```python
from build123d import *

# Parameters (mm, degrees)
BOSS_EXTRUDE1_START = -9
SKETCH2_R           = 10
BOSS_EXTRUDE1_DEPTH = 1


with BuildPart() as part:
    # Sketch1 → Revolve1 (revolve)
    with BuildSketch(Plane.XY, mode=Mode.PRIVATE) as revolve1_sk:
        Polygon((0.905904645, 10.418424893), (2.905904645, 10.418424893), (2.905904645, 0.418424893), (9.905904645, 0.418424893), (9.905904645, -1.581575107), (0.905904645, -1.581575107), (0.905904645, 8.418424893), align=None)
    revolve(revolve1_sk.sketch.rotate(Axis((0.905904645, -9.581575107, 0), (1, 0, 0)), 90), axis=Axis((0.905904645, -9.581575107, 0), (1, 0, 0)))

    # Sketch2 → Boss-Extrude1 (add)
    with BuildSketch(Plane(origin=(9.905904645, 0, 0), x_dir=(0, 0, -1), z_dir=(1, 0, 0)).offset(BOSS_EXTRUDE1_START)):
        with Locations(Location((0, -9.581575107, 0), (0, 0, 180))):
            Circle(SKETCH2_R)
    extrude(amount=BOSS_EXTRUDE1_DEPTH)


solid = part.part
```
Geometry: final body of the model. Coordinates: model frame, mm. A direction names the side the tool comes from. Coordinates: 2 decimals unless noted, no trailing zeros. Write each loop counter-clockwise with the first axis right and the second up, starting at its lowest first coordinate (ties: lowest second). Pieces come first, ordered by that corner, then holes. Notation, with made-up numbers: M 35.25,-24.5 L 76.25,-24.5 A20 ccw 76.25,-17.5 Z; hole C 26.5,89.25 d3. An arc over 180 degrees is marked long. Answer as CSV lines item,"result". Start each with the question number.
Q1. Cut plane A-A on z = 0. Return the cut outline in (x, y).
Q2. Reachability of faces 5 (the flat face through (2.906, -19, 4)), 6 (the flat face through (0.906, -10, 0)) from +Z, -Z, +X, -X, +Y, -Y: full face, straight path, thin tool, end or side. Return the list, or none.
Q3. Cut plane B-B on y = -3. Return the cut outline in (x, z).
Q4. Line query: line 1 (Y direction, x = 5.25, z = 0); line 2 (X direction, y = -27, z = 1.5); line 3 (Z direction, x = 8.25, y = -2.5). Output: solid intervals per line, ascending. Write a range as from..to.
Q5. Cut plane D-D on z = -12.5. Return the cut outline in (x, y).
Q6. Cut plane C-C on x = 7.5. Return the cut outline in (y, z).
Q7. Pin query (flat end, axial travel): P1, Ø1, axis at x = 7, z = -3, coming from the -Y side; P2, Ø5, axis at x = 7, y = -21, coming from the -Z side; P3, Ø4, axis at x = 7, z = -1.5, coming from the +Y side. Return the tip coordinate at first contact, or that it passes through.
Q8. Mould query, pull axis Z, two halves, no side actions, for faces 1 (the cylindrical face through (6.45, -3.5, -7.94)), 2 (the cylindrical face through (5.85, -17.513, -1.041)), 3 (the flat face through (9.906, -18, 0)), 4 (the flat face through (1.906, -10, 0)). Classes: released by +Z, released by -Z, zero draft, split by the parting line, or undercut.
Findings below:
1,outline,"M 0.91,-29.58 L 2.91,-29.58 L 2.91,-19.58 L 9.91,-19.58 L 9.91,-17.58 L 1.91,-17.58 L 1.91,-1.58 L 9.91,-1.58 L 9.91,0.42 L 2.91,0.42 L 2.91,10.42 L 0.91,10.42 Z"
2,face 5,"+X"
2,face 6,"+Z, -Z, -X, +Y, -Y"
3,outline,"M 0.91,-18.89 L 2.91,-18.89 L 2.91,-7.53 L 9.91,-7.53 L 9.91,-4.55 L 1.91,-4.55 L 1.91,4.55 L 9.91,4.55 L 9.91,7.53 L 2.91,7.53 L 2.91,18.89 L 0.91,18.89 Z"
4,line 1,"y = -19.58..-17.58, -1.58..0.42"
4,line 2,"x = 0.91..2.91"
4,line 3,"z = -7.06..-3.72, 3.72..7.06"
5,outline,"M 0.91,-25.19 L 2.91,-25.19 L 2.91,6.03 L 0.91,6.03 Z"
6,outline,"C -9.58,0 d20; hole C -9.58,0 d16"
7,P1,"stops at y = -19.26"
7,P2,"stops at z = -4.52"
7,P3,"stops at y = 0.42"
8,face 1,"split by the parting line"
8,face 2,"undercut"
8,face 3,"zero draft"
8,face 4,"undercut"
